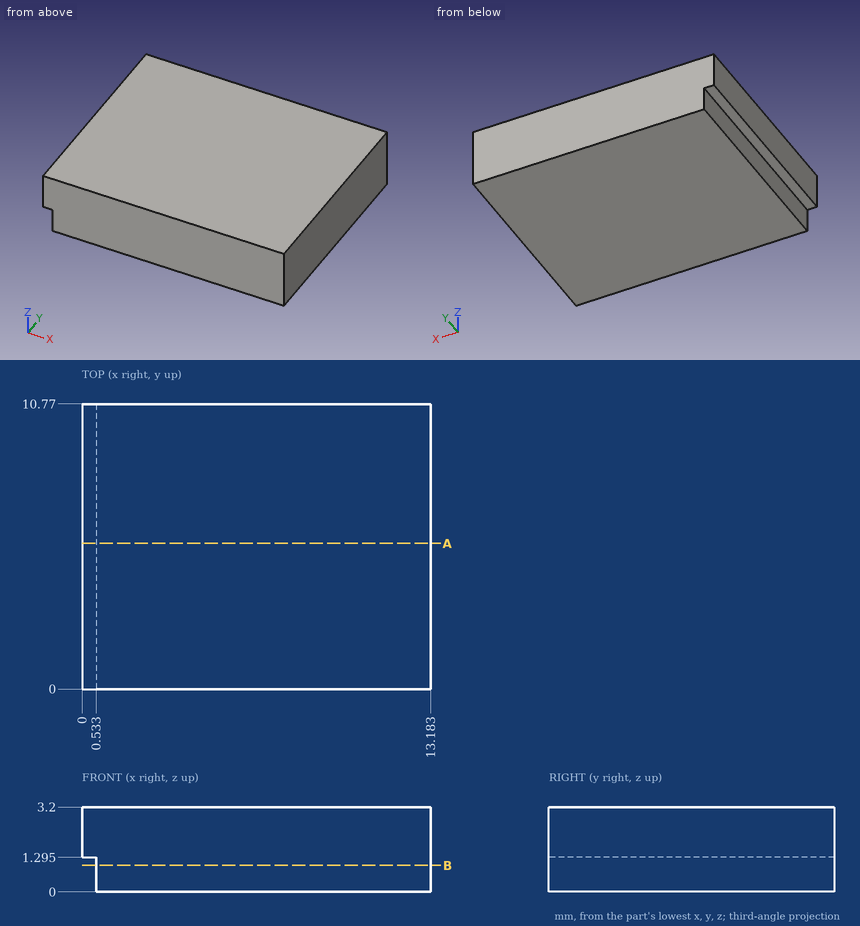
Design review of the part shown in the three views and the two pictorial views. Dimensions are in mm from the part's minimum x, y and z. Round coordinates to 2 decimals unless told otherwise and drop trailing zeros. Loops run counter-clockwise (first coordinate to the right, second up) from the corner with the lowest first, then second, coordinate; pieces in that order, holes last. Notation, with made-up numbers: M 82,-7 L 130,-7 A13 cw 130,2 Z; hole C 73,-37 d10. An arc over 180 degrees is marked long. Put each result on its own line as item: value.
Q1. Consider section B-B, the plane z = 1. Give the boundary of the cut face in (x, y), then the cut area to 3 significant figures.
Result set:
outline: M 0.53,0 L 13.18,0 L 13.18,10.77 L 0.53,10.77 Z
area: 136 mm²
Q2. For pin 1 (1 mm diameter, centred on y = 5.5, z = 0.5, fed in from -X), flat-tipped, find the tip position at first contact; note if it passes through.
Result set:
pin 1: stops at x = 0.53
Q3. To check wall thickness, follow L1, parallel to X at y = 7, z = 1.25. State the ranges of the line that lie inside material, in increasing order.
Result set:
L1: x = 0.53 to 13.18
Q4. Consider section A-A, the plane y = 5.5. Give the boundary of the cut face in (x, z) (1 decimal).
Result set:
outline: M 0,1.3 L 0.5,1.3 L 0.5,0 L 13.2,0 L 13.2,3.2 L 0,3.2 Z
